Answer from the drawing. Dimensions are ordinates in mm from the lowest x, y and z of the part. Coordinates: 2 decimals unless noted, no trailing zeros. Write each loop counter-clockwise with the first axis right and the second up, starting at its lowest first coordinate (ties: lowest second). Pieces come first, ordered by that corner, then holes. Notation, with made-up numbers: (72, 89.5) - (79, 89.5) arc R13 ccw to (79, 106.5) - close; hole circle Ø9 at (86, 27.25). An arc over 180 degrees is marked (long way). Use a Markdown table: item, result.
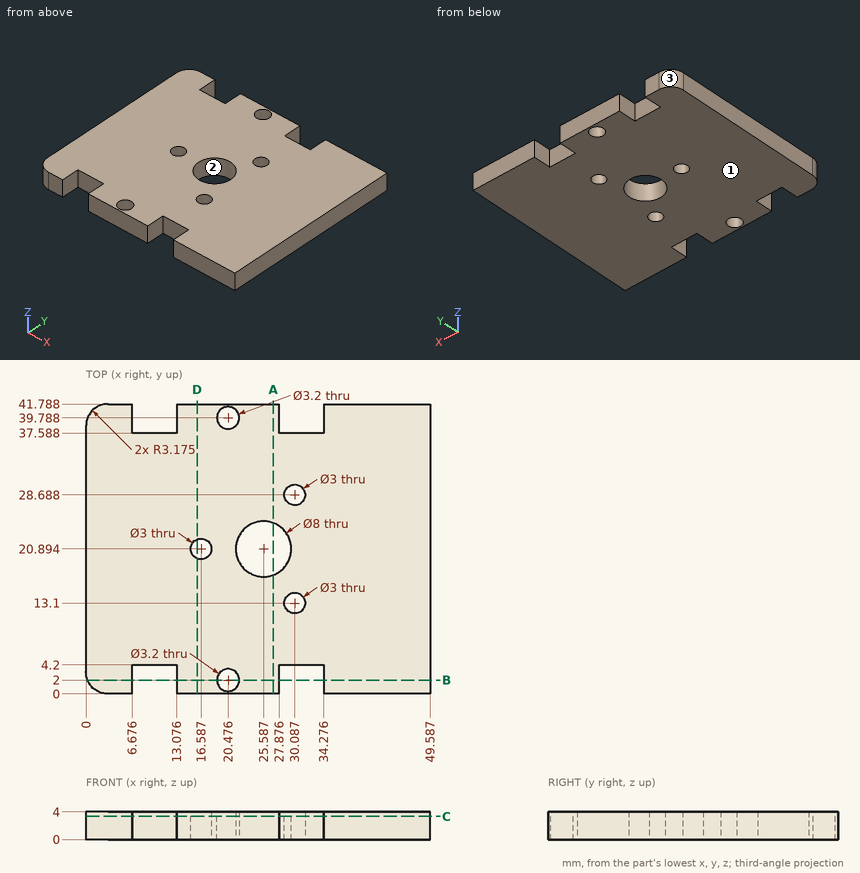
(1) A cutting plane is placed at C-C, the plane z = 3.35. Count the separate pieces of the cut face and the enclosed holes in it, and give its area (3 significant figures).
Report:
| item | result |
|---|---|
| separate pieces | 1 |
| enclosed holes | 6 |
| area | 1,870 mm² |
(2) A cutting plane is placed at D-D, the plane x = 16. Write down the section's boundary in (y, z) (1 decimal), and give its area (3 significant figures).
Report:
| item | result |
|---|---|
| outline | (0, 0) - (19.5, 0) - (19.5, 4) - (0, 4) - close; (22.3, 0) - (41.8, 0) - (41.8, 4) - (22.3, 4) - close |
| area | 156 mm² |
(3) The mould has two halves that part along X. Classify the marked faces 1, 2 and 3: pulls with the +X half, pulls with the -X half, needs draft (parallel to the pull), parting line crosses it, or undercut.
Report:
| item | result |
|---|---|
| face 1 | needs draft |
| face 2 | undercut |
| face 3 | pulls with the -X half |
(4) A cutting plane is placed at B-B, the plane y = 2. Write down the section's boundary in (x, z) (1 decimal).
Report:
| item | result |
|---|---|
| outline | (0.2, 0) - (6.7, 0) - (6.7, 4) - (0.2, 4) - close; (13.1, 0) - (18.9, 0) - (18.9, 4) - (13.1, 4) - close; (22.1, 0) - (27.9, 0) - (27.9, 4) - (22.1, 4) - close; (34.3, 0) - (49.6, 0) - (49.6, 4) - (34.3, 4) - close |
(5) Each of these flat-tipped pins is pushed along its axis until it touches: P1, Ø1.5, axis at y = 4.5, z = 3, coming from the -X side; P2, Ø1.2, axis at x = 32, z = 2, coming from the +Y side. Where does it stop, or does it pass through?
Report:
| item | result |
|---|---|
| P1 | stops at x = 0 |
| P2 | stops at y = 37.59 |
(6) A cutting plane is placed at A-A, the plane x = 27. Write down the section's boundary in (y, z).
Report:
| item | result |
|---|---|
| outline | (0, 0) - (17.15, 0) - (17.15, 4) - (0, 4) - close; (24.64, 0) - (41.79, 0) - (41.79, 4) - (24.64, 4) - close |
(7) Straight lines are drawn through the part: L1, parallel to X at y = 38.5, z = 3 (1 decimal); L2, parallel to Y at x = 3, z = 3.15 (1 decimal); L3, parallel to Y at x = 10.5, z = 1.7. For each, find the intervals that lie inside material, in ascending order.
Report:
| item | result |
|---|---|
| L1 | x = 0 to 6.7, 13.1 to 19.5, 21.4 to 27.9, 34.3 to 49.6 |
| L2 | y = 0 to 41.8 |
| L3 | y = 4.2 to 37.59 |
